For this review, use the dimensioned drawing (mm, ordinates from the lowest corner) and the shaded views. A direction names the side the tool comes from. Coordinates: 2 decimals unless noted, no trailing zeros. Loops run counter-clockwise (first coordinate to the right, second up) from the corner with the lowest first, then second, coordinate; pieces in that order, holes last. Notation, with made-up numbers: (29.5, 40) - (55.5, 40) arc R16 ccw to (55.5, 62) - close; hole circle Ø9 at (78, 58). An arc over 180 degrees is marked (long way). Answer in a Markdown table with one row per item. Add a question column.
(1) We need section B-B, the plane y = 11.5. Write out the cut boundary in (x, z), plus the area to 3 significant figures.
(2) To check wall thickness, follow L1, parallel to X at y = 8, z = 87; L2, parallel to Z at x = 56.5, y = 12.75; L3, parallel to X at y = 8, z = 124.5 (1 decimal). State the ranges of each line that lie inside material, in increasing order. Write a range as [from, to].
(3) For the marked faces 1, 2, 3, 4 and 5, list the 3-axis set-ups (+Z, -Z, +X, -X, +Y, -Y) from which the entire face can be reached by the end or side of a thin tool; tool diameter is ignored.
(4) We need section D-D, the plane z = 111.5. Write out the cut boundary in (x, y).
(5) We need section C-C, the plane z = 70.5. Write out the cut boundary in (x, y), plus the area to 3 significant figures.
(6) We need section A-A, the plane x = 50.5. Write out the cut boundary in (y, z).
(7) The part is to be moulded in two halves that separate along Z. For the marked faces 6, 7 and 8, say which applies: released by +Z, released by -Z, zero draft, split by the parting line, or undercut.
(8) Clearance check with flat-ended pins moving along their axes: pin 1 (10 mm diameter, centred on y = 11, z = 74, fed in from +X); pin 2 (1.2 mm diameter, centred on x = 90.5, y = 1, fed in from -Z); pin 3 (1.5 mm diameter, centred on x = 58.5, z = 69.5, fed in from +Y). State where each tip first meets the part, or that it passes through.
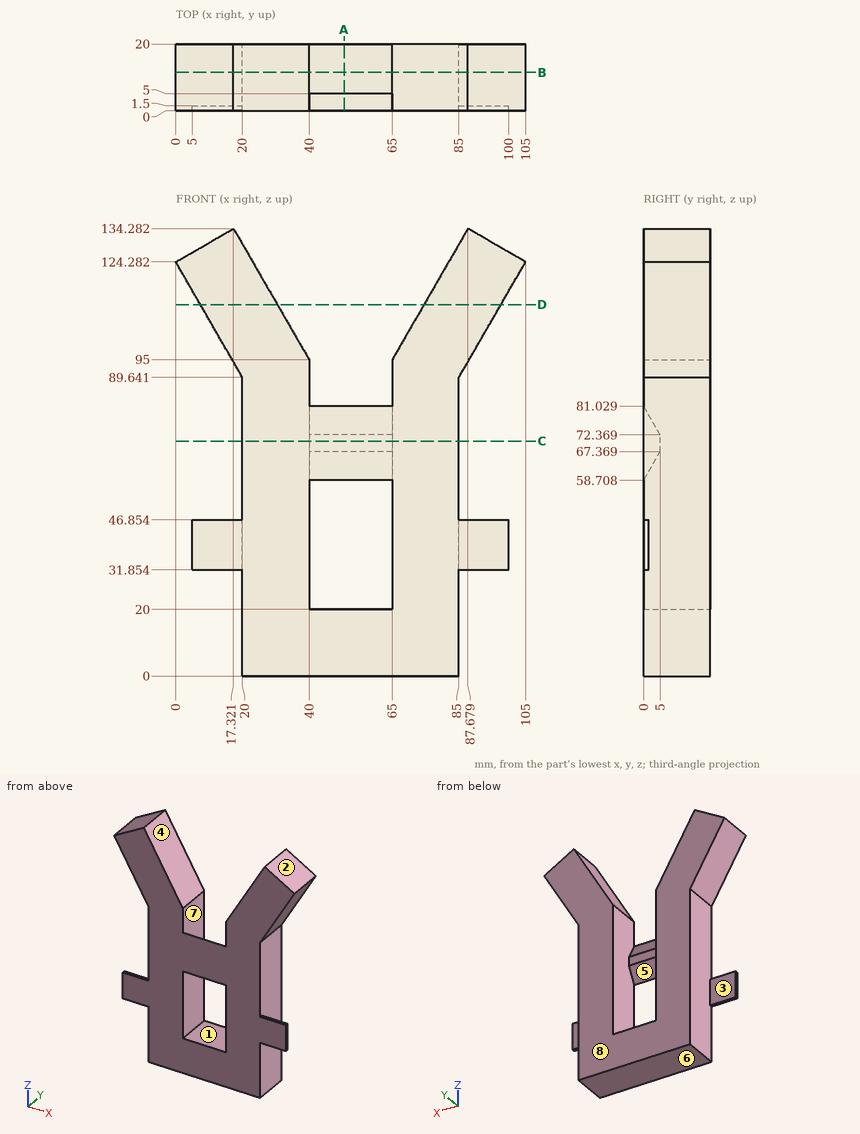
Responses:
| question | item | result |
|---|---|---|
| 1 | outline | (0, 124.28) - (20, 89.64) - (20, 0) - (85, 0) - (85, 89.64) - (105, 124.28) - (87.68, 134.28) - (65, 95) - (65, 20) - (40, 20) - (40, 95) - (17.32, 134.28) - close |
| 1 | area | 5,900 mm2 |
| 2 | L1 | x = [20, 40], [65, 85] |
| 2 | L2 | z = [0, 20] |
| 2 | L3 | x = [0.4, 23], [82, 104.6] |
| 3 | face 1 | +Y, -Y |
| 3 | face 2 | +Z, +X, +Y, -Y |
| 3 | face 3 | -Z, -X, +Y |
| 3 | face 4 | +Z, +Y, -Y |
| 3 | face 5 | +Y |
| 4 | outline | (7.38, 0) - (30.47, 0) - (30.47, 20) - (7.38, 20) - close; (74.53, 0) - (97.62, 0) - (97.62, 20) - (74.53, 20) - close |
| 5 | outline | (20, 0) - (85, 0) - (85, 20) - (65, 20) - (65, 5) - (40, 5) - (40, 20) - (20, 20) - close |
| 5 | area | 925 mm2 |
| 6 | outline | (0, 0) - (20, 0) - (20, 20) - (0, 20) - close; (0, 58.71) - (5, 67.37) - (5, 72.37) - (0, 81.03) - close |
| 7 | face 6 | released by -Z |
| 7 | face 7 | undercut |
| 7 | face 8 | zero draft |
| 8 | pin 1 | stops at x = 85 |
| 8 | pin 2 | stops at z = 31.85 |
| 8 | pin 3 | stops at y = 5 |
